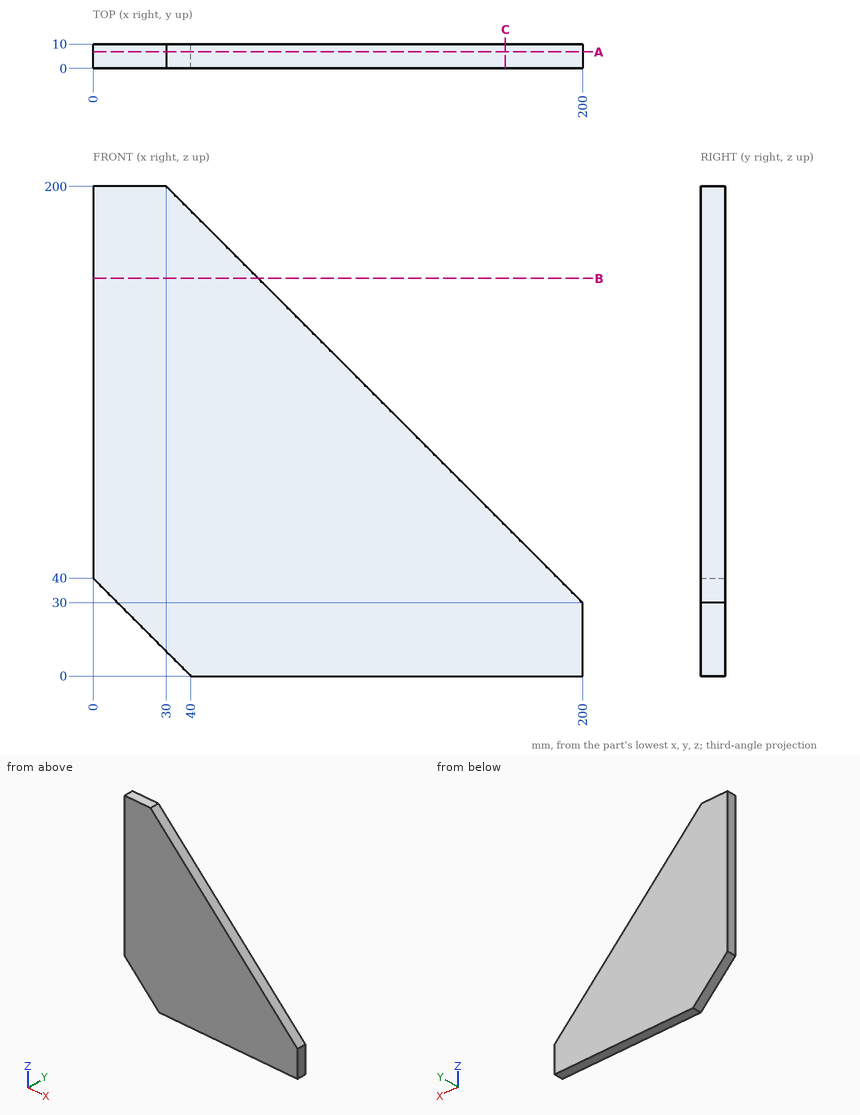
Here's the drawing with two shaded views (mm, measured from the low corner). I have some questions. Coordinates: 2 decimals unless noted, no trailing zeros. Loops run counter-clockwise (first coordinate to the right, second up) from the corner with the lowest first, then second, coordinate; pieces in that order, holes last. Notation, with made-up numbers: (-4, 74) -> (18, 74) arc R29 cw to (18, 108) -> close; hole circle Ø3 at (-13.5, 86.25). An arc over 180 degrees is marked (long way). Put each result on its own line as item: value. Start each with the question number.
Q1. I want a section at C-C (x = 168.5). Write out the boundary of the cut face in (y, z).
Q2. If I drill on line 1 (Z direction, x = 30, y = 2); line 2 (Z direction, x = 134, y = 5.75); line 3 (X direction, y = 5.5, z = 143.5), over which ranges is the centre line in solid material (lowest first)? Write a range as [from, to].
Q3. I want a section at B-B (z = 162.5). Write out the boundary of the cut face in (x, y), plus the area to 3 significant figures.
Q4. I'm going to push flat-ended pins straight in: P1, Ø3, axis at y = 5, z = 157.5, coming from the +X side; P2, Ø4, axis at y = 7.5, z = 38.5, coming from the +X side; P3, Ø3, axis at y = 8.5, z = 33, coming from the -X side. Where does each tip first touch, or does it pass through?
Q5. I want a section at A-A (y = 6.75). Write out the boundary of the cut face in (x, z), plus the area to 4 significant figures.
Taken from the geometry:
1. outline: (0, 0) -> (10, 0) -> (10, 61.5) -> (0, 61.5) -> close
2. line 1: z = [10, 200]
2. line 2: z = [0, 96]
2. line 3: x = [0, 86.5]
3. outline: (0, 0) -> (67.5, 0) -> (67.5, 10) -> (0, 10) -> close
3. area: 675 mm2
4. P1: stops at x = 74
4. P2: stops at x = 193.5
4. P3: stops at x = 5.5
5. outline: (0, 40) -> (40, 0) -> (200, 0) -> (200, 30) -> (30, 200) -> (0, 200) -> close
5. area: 24,750 mm2
